The figure shows three views and two pictorial views of one solid part (mm, origin at its lowest corner). Answer the questions. A direction names the side the tool comes from. Give positions to 0.01 mm unless a question says otherwise; leave off trailing zeros. Loops run counter-clockwise (first coordinate to the right, second up) from the corner with the lowest first, then second, coordinate; pieces in that order, holes last.
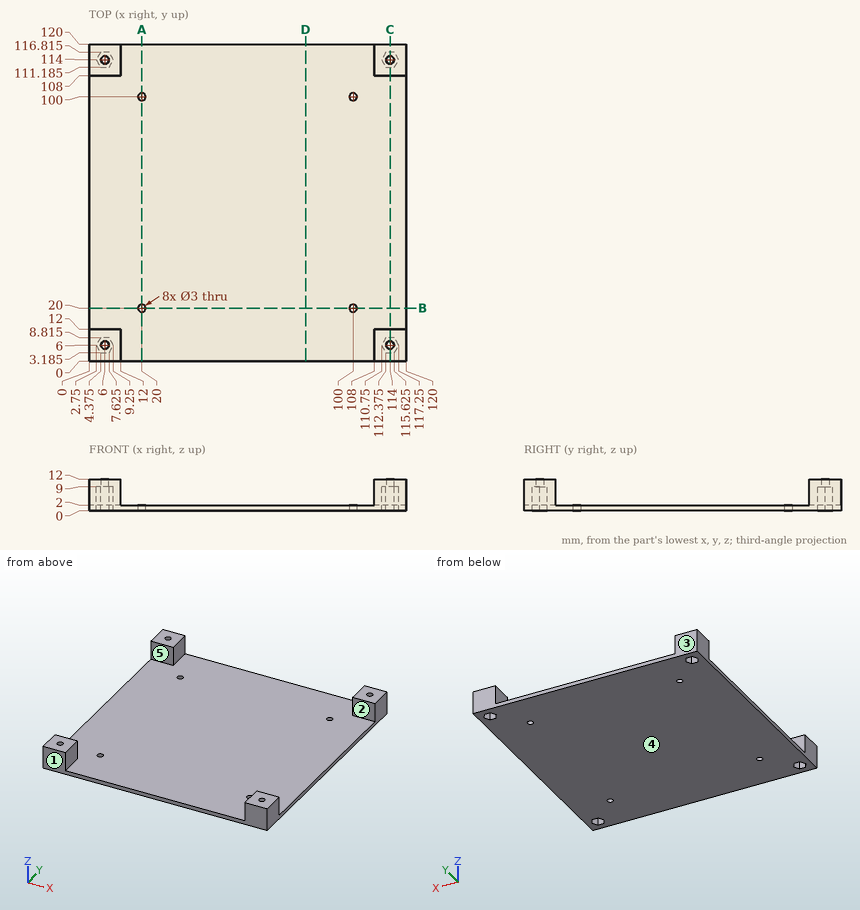
Q1. Which of the six approach directions +Z, -Z, +X, -X, +Y, -Y give full straight-line access (tool end or side, diameter ignored) to the marked faces 1 and 2?
Q2. Section A-A on x = 20 is taken. Give the vertices of the cut face in (y, z), plus the area to 3 significant figures.
Q3. Given pin 1 (6 mm diameter, centred on x = 97.5, y = 64.5, fed in from +Z); pin 2 (4 mm diameter, centred on x = 114, y = 114, fed in from -Z), each flat-ended and moving along its own axis, determine where each tip first touches the part or whether it passes through.
Q4. Section D-D on x = 82 is taken. Give the vertices of the cut face in (y, z), plus the area to 3 significant figures.
Q5. Consider line 1 along X through (y, z) = (114, 10.5); line 2 along Y through (x, z) = (100, 1.5). Determine where each line is inside the solid, lowest interval first.
Q6. Section C-C on x = 114 is taken. Give the vertices of the cut face in (y, z) (1 decimal).
Q7. Determine the mould class of the marked faces 3, 4 and 5 for opening direction Y: +Y half, -Y half, draft (parallel to the pull), parting line (faces both ways), or undercut.
Check result:
1. face 1: +Z, -Z, +X, -X, -Y
1. face 2: +Z, +X, -X
2. outline: (0, 0) - (18.5, 0) - (18.5, 2) - (0, 2) - close; (21.5, 0) - (98.5, 0) - (98.5, 2) - (21.5, 2) - close; (101.5, 0) - (120, 0) - (120, 2) - (101.5, 2) - close
2. area: 228 mm2
3. pin 1: stops at z = 2
3. pin 2: stops at z = 9
4. outline: (0, 0) - (120, 0) - (120, 2) - (0, 2) - close
4. area: 240 mm2
5. line 1: x = 0 to 4.5, 7.5 to 12, 108 to 112.5, 115.5 to 120
5. line 2: y = 0 to 18.5, 21.5 to 98.5, 101.5 to 120
6. outline: (0, 0) - (3.2, 0) - (3.2, 9) - (4.5, 9) - (4.5, 12) - (0, 12) - close; (7.5, 9) - (8.8, 9) - (8.8, 0) - (111.2, 0) - (111.2, 9) - (112.5, 9) - (112.5, 12) - (108, 12) - (108, 2) - (12, 2) - (12, 12) - (7.5, 12) - close; (115.5, 9) - (116.8, 9) - (116.8, 0) - (120, 0) - (120, 12) - (115.5, 12) - close
7. face 3: +Y half
7. face 4: draft
7. face 5: undercut
